from build123d import *

# Parameters (mm, degrees)
BOSS_EXTRUDE1_DEPTH = 17.85
SKETCH5_R           = 1
CUT_EXTRUDE1_DEPTH  = 10
SKETCH6_W           = 34.25
SKETCH6_H           = 9
BOSS_EXTRUDE2_DEPTH = 3
SKETCH7_W           = 17.85
SKETCH7_H           = 15.1
BOSS_EXTRUDE3_DEPTH = 5.225
BOSS_EXTRUDE4_START = 23.25
SKETCH7_3_W         = 17.85
SKETCH7_3_H         = 15.1
BOSS_EXTRUDE4_DEPTH = 5.225
CUT_EXTRUDE2_REACH  = 125.33
SKETCH8_W           = 7.725
SKETCH8_H           = 18
SKETCH9_W           = 34.25
SKETCH9_H           = 3
BOSS_EXTRUDE5_DEPTH = 18
SKETCH10_W          = 12.8
SKETCH10_H          = 2.9
CUT_EXTRUDE3_DEPTH  = 14.85
CUT_EXTRUDE4_REACH  = 124.932
SKETCH11_W          = 7.725
SKETCH11_H          = 18
SKETCH12_W          = 18.8
SKETCH12_H          = 18
CUT_EXTRUDE5_DEPTH  = 4.45
SKETCH13_W          = 18.8
SKETCH13_H          = 18
BOSS_EXTRUDE6_DEPTH = 3


with BuildPart() as part:
    # Sketch4 → Boss-Extrude1 (new body)
    with BuildSketch(Plane(origin=(0, 0, -70.608208955), x_dir=(-1, 0, 0), z_dir=(0, 0, -1))):
        Polygon((-69.066917791, 81.5), (-45.816917791, 81.5), (-45.816917791, 96.6), (-40.316917791, 96.6), (-40.316917791, 78.6), (-74.566917791, 78.6), (-74.566917791, 96.6), (-69.066917791, 96.6), align=None)
    extrude(amount=BOSS_EXTRUDE1_DEPTH)

    # Sketch5 → Cut-Extrude1 (cut)
    with BuildSketch(Plane(origin=(0, 0, -88.458208955), x_dir=(-1, 0, 0), z_dir=(0, 0, -1))):
        with Locations((-43.741917791, 88)):
            Circle(SKETCH5_R)
        with Locations((-71.141917791, 88)):
            Circle(SKETCH5_R)
    extrude(amount=-CUT_EXTRUDE1_DEPTH, mode=Mode.SUBTRACT)

    # Sketch6 → Boss-Extrude2 (add)
    with BuildSketch(Plane(origin=(0, 0, -70.608208955), x_dir=(-1, 0, 0), z_dir=(0, 0, -1))):
        with Locations((-57.441917791, 74.1)):
            Rectangle(SKETCH6_W, SKETCH6_H)
        with BuildLine():
            Line((-68.111940299, 77.5), (-44.896828216, 77.5))
            ThreePointArc((-44.896828216, 77.5), (-42.396828216, 75), (-44.896828216, 72.5))
            Line((-44.896828216, 72.5), (-68.111940299, 72.5))
            ThreePointArc((-68.111940299, 72.5), (-70.611940299, 75), (-68.111940299, 77.5))
        make_face(mode=Mode.SUBTRACT)
    extrude(amount=BOSS_EXTRUDE2_DEPTH)

    # Sketch7 → Boss-Extrude3 (add)
    with BuildSketch(Plane(origin=(45.816917791, 0, 0), x_dir=(0, 0, -1), z_dir=(1, 0, 0))):
        with Locations((79.533208955, 89.05)):
            Rectangle(SKETCH7_W, SKETCH7_H)
    extrude(amount=BOSS_EXTRUDE3_DEPTH)

    # Sketch7<3> → Boss-Extrude4 (add)
    with BuildSketch(Plane(origin=(45.816917791, 0, 0), x_dir=(0, 0, -1), z_dir=(1, 0, 0)).offset(BOSS_EXTRUDE4_START)):
        with Locations((79.533208955, 89.05)):
            Rectangle(SKETCH7_3_W, SKETCH7_3_H)
    extrude(amount=-BOSS_EXTRUDE4_DEPTH)

    # Sketch8 → Cut-Extrude2 (cut, up to next)
    with BuildSketch(Plane(origin=(0, 0, -88.458208955), x_dir=(-1, 0, 0), z_dir=(0, 0, -1)), mode=Mode.PRIVATE) as cut_extrude2_sk1:
        with Locations((-70.704417791, 87.6)):
            Rectangle(SKETCH8_W, SKETCH8_H)
    cut_extrude2_tool1 = extrude(cut_extrude2_sk1.sketch, amount=-CUT_EXTRUDE2_REACH, mode=Mode.PRIVATE) & part.part
    # Sketch8 → Cut-Extrude2 (cut, up to next)
    with BuildSketch(Plane(origin=(0, 0, -88.458208955), x_dir=(-1, 0, 0), z_dir=(0, 0, -1)), mode=Mode.PRIVATE) as cut_extrude2_sk2:
        with Locations((-44.179417791, 87.6)):
            Rectangle(SKETCH8_W, SKETCH8_H)
    cut_extrude2_tool2 = extrude(cut_extrude2_sk2.sketch, amount=-CUT_EXTRUDE2_REACH, mode=Mode.PRIVATE) & part.part
    add(cut_extrude2_tool1.solids().sort_by_distance((70.704418, 87.6, -88.458209))[0], mode=Mode.SUBTRACT)
    add(cut_extrude2_tool2.solids().sort_by_distance((44.179418, 87.6, -88.458209))[0], mode=Mode.SUBTRACT)

    # Sketch9 → Boss-Extrude5 (add)
    with BuildSketch(Plane(origin=(0, 78.6, 0), x_dir=(1, 0, 0), z_dir=(0, 1, 0))):
        with Locations((57.441917791, 72.108208955)):
            Rectangle(SKETCH9_W, SKETCH9_H)
    extrude(amount=BOSS_EXTRUDE5_DEPTH)

    # Sketch10 → Cut-Extrude3 (cut)
    with BuildSketch(Plane(origin=(0, 0, -88.458208955), x_dir=(-1, 0, 0), z_dir=(0, 0, -1))):
        with Locations((-57.441917791, 80.05)):
            Rectangle(SKETCH10_W, SKETCH10_H)
    extrude(amount=-CUT_EXTRUDE3_DEPTH, mode=Mode.SUBTRACT)

    # Sketch11 → Cut-Extrude4 (cut, up to next)
    with BuildSketch(Plane(origin=(0, 0, -73.608208955), x_dir=(-1, 0, 0), z_dir=(0, 0, -1)), mode=Mode.PRIVATE) as cut_extrude4_sk1:
        with Locations((-70.704417791, 87.6)):
            Rectangle(SKETCH11_W, SKETCH11_H)
    cut_extrude4_tool1 = extrude(cut_extrude4_sk1.sketch, amount=-CUT_EXTRUDE4_REACH, mode=Mode.PRIVATE) & part.part
    # Sketch11 → Cut-Extrude4 (cut, up to next)
    with BuildSketch(Plane(origin=(0, 0, -73.608208955), x_dir=(-1, 0, 0), z_dir=(0, 0, -1)), mode=Mode.PRIVATE) as cut_extrude4_sk2:
        with Locations((-44.179417791, 87.6)):
            Rectangle(SKETCH11_W, SKETCH11_H)
    cut_extrude4_tool2 = extrude(cut_extrude4_sk2.sketch, amount=-CUT_EXTRUDE4_REACH, mode=Mode.PRIVATE) & part.part
    add(cut_extrude4_tool1.solids().sort_by_distance((70.704418, 87.6, -73.608209))[0], mode=Mode.SUBTRACT)
    add(cut_extrude4_tool2.solids().sort_by_distance((44.179418, 87.6, -73.608209))[0], mode=Mode.SUBTRACT)

    # Sketch12 → Cut-Extrude5 (cut)
    with BuildSketch(Plane(origin=(0, 0, -88.458208955), x_dir=(-1, 0, 0), z_dir=(0, 0, -1))):
        with Locations((-57.441917791, 87.6)):
            Rectangle(SKETCH12_W, SKETCH12_H)
    extrude(amount=-CUT_EXTRUDE5_DEPTH, mode=Mode.SUBTRACT)

    # Sketch13 → Boss-Extrude6 (add)
    with BuildSketch(Plane(origin=(0, 0, -84.008208955), x_dir=(-1, 0, 0), z_dir=(0, 0, -1))):
        with Locations((-57.441917791, 87.6)):
            Rectangle(SKETCH13_W, SKETCH13_H)
    extrude(amount=BOSS_EXTRUDE6_DEPTH)


solid = part.part
Read the model definition and answer for the solid it produces. Units are mm, in the model's axes. A direction names the side the tool comes from. Round coordinates to 2 decimals unless told otherwise and drop trailing zeros. Write each loop counter-clockwise with the first axis right and the second up, starting at its lowest first coordinate (ties: lowest second). Pieces come first, ordered by that corner, then holes.
Q1. Find section B-B on y = 75. Determine the outline of the cut face in (x, z), and give its area (3 significant figures).
Values:
outline: (40.32, -73.61) - (42.4, -73.61) - (42.4, -70.61) - (40.32, -70.61) - close; (70.61, -73.61) - (74.57, -73.61) - (74.57, -70.61) - (70.61, -70.61) - close
area: 18.1 mm2
Q2. Find section C-C on y = 89. Determine the outline of the cut face in (x, z), and give its area (3 significant figures).
Values:
outline: (48.04, -87.01) - (66.84, -87.01) - (66.84, -70.61) - (48.04, -70.61) - close; hole (51.04, -84.01) - (63.84, -84.01) - (63.84, -73.61) - (51.04, -73.61) - close
area: 175 mm2
Q3. A tool of negligible diameter and unlimited length cuts with its end or side. For faces 4 (the face through (56, 72.5, -72)), 5 (the face through (51.042, 88, -79)), 6 (the face through (44, 78.6, -72)), from which of +Z, -Z, +X, -X, +Y, -Y can it reach the whole face along a straight path? Write none if from no direction.
Values:
face 4: +Z, -Z
face 5: +Y, -Y
face 6: +Z, -Z, -X, +Y
Q4. The mould has two halves that part along X. Classify faces 1 (the face through (74.567, 74, -72)), 2 (the face through (58, 78.6, -85)), 3 (the face through (42.4, 75.1, -72.1)): released by +X, released by -X, zero draft, split by the parting line, or undercut.
Values:
face 1: released by +X
face 2: zero draft
face 3: undercut
Q5. Find section A-A on x = 47. Determine the outline of the cut face in (y, z).
Values:
outline: (69.6, -73.61) - (72.5, -73.61) - (72.5, -70.61) - (69.6, -70.61) - close; (77.5, -73.61) - (78.6, -73.61) - (78.6, -70.61) - (77.5, -70.61) - close
Q6. Find section D-D on x = 54.5. Determine the outline of the cut face in (y, z), and give its area (3 significant figures).
Values:
outline: (69.6, -73.61) - (72.5, -73.61) - (72.5, -70.61) - (69.6, -70.61) - close; (77.5, -73.61) - (96.6, -73.61) - (96.6, -70.61) - (77.5, -70.61) - close; (78.6, -87.01) - (96.6, -87.01) - (96.6, -84.01) - (78.6, -84.01) - close
area: 120 mm2
Q7. Flat-ended cylindrical pins translate along their axes: P1, Ø8.5, axis at y = 91, z = -78.5, coming from the +X side; P2, Ø5, axis at y = 80.5, z = -83, coming from the -X side; P3, Ø2, axis at x = 65, z = -84, coming from the -Y side. Find the tip coordinate at first contact, or state that the pin passes through.
Values:
P1: stops at x = 66.84
P2: stops at x = 48.04
P3: stops at y = 78.6
Q8. Straight lines are drawn through the part: line 1 (Y direction, x = 49.5, z = -71.5); line 2 (X direction, y = 85.75, z = -82.5); line 3 (Z direction, x = 54, y = 90.5). For each, find the intervals that lie inside material, in ascending order.
Values:
line 1: y = 69.6 to 72.5, 77.5 to 96.6
line 2: x = 48.04 to 51.04, 63.84 to 66.84
line 3: z = -87.01 to -84.01, -73.61 to -70.61
